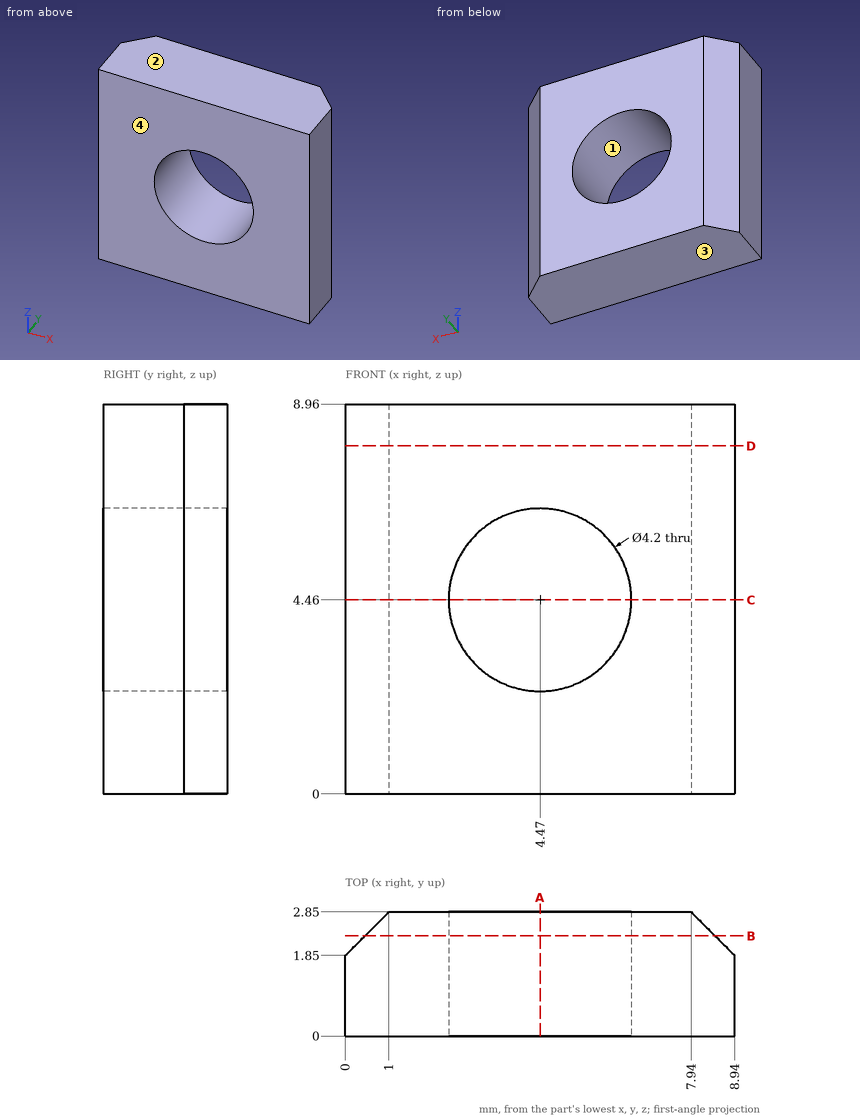
Answer from the drawing. Dimensions are ordinates in mm from the lowest x, y and z of the part. Round coordinates to 2 decimals unless told otherwise and drop trailing zeros. Loops run counter-clockwise (first coordinate to the right, second up) from the corner with the lowest first, then second, coordinate; pieces in that order, holes last.
Q1. Section A-A on x = 4.47 is taken. Write down the section's boundary in (y, z).
Q2. Section B-B on y = 2.3 is taken. Write down the section's boundary in (x, z).
Q3. Section D-D on z = 8 is taken. Write down the section's boundary in (x, y), and give its area (3 significant figures).
Q4. Consider probe 1 along Z at (x, y) = (4.47, 1.7); probe 2 along Z at (x, y) = (5, 0.2); probe 3 along X at (y, z) = (2.75, 4.25). Determine where each line is inside the solid, lowest interval first.
Q5. Section C-C on z = 4.46 is taken. Write down the section's boundary in (x, y).
Q6. Determine the mould class of the marked faces 1, 2, 3 and 4 for opening direction Z: released by +Z, released by -Z, zero draft, split by the parting line, or undercut.
Output:
1. outline: (0, 0) - (2.85, 0) - (2.85, 2.36) - (0, 2.36) - close; (0, 6.56) - (2.85, 6.56) - (2.85, 8.96) - (0, 8.96) - close
2. outline: (0.45, 0) - (8.49, 0) - (8.49, 8.96) - (0.45, 8.96) - close; hole circle Ø4.2 at (4.47, 4.46)
3. outline: (0, 0) - (8.94, 0) - (8.94, 1.85) - (7.94, 2.85) - (1, 2.85) - (0, 1.85) - close
3. area: 24.5 mm2
4. probe 1: z = 0 to 2.36, 6.56 to 8.96
4. probe 2: z = 0 to 2.43, 6.49 to 8.96
4. probe 3: x = 0.9 to 2.38, 6.56 to 8.04
5. outline: (0, 0) - (2.37, 0) - (2.37, 2.85) - (1, 2.85) - (0, 1.85) - close; (6.57, 0) - (8.94, 0) - (8.94, 1.85) - (7.94, 2.85) - (6.57, 2.85) - close
6. face 1: undercut
6. face 2: released by +Z
6. face 3: released by -Z
6. face 4: zero draft
